Autodesk Inventor part; units mm, degrees
ref_plane "YZ Plane" through (0, 0, 0) normal (1, 0, 0) x (0, 1, 0)
ref_plane "XZ Plane" through (0, 0, 0) normal (0, 1, 0) x (-1, 0, 0)
ref_plane "XY Plane" through (0, 0, 0) normal (0, 0, 1) x (1, 0, 0)
sketch "Sketch1" plane through (0, 0, 0) normal (0, 0, 1) x (1, 0, 0)
  line L0 (34.925, 0) -> (34.925, 12.7)
  arc A0 (34.925, 53.1813) -> (0, 76.2) centre (2.0699, 41.3364) ccw
  line L1 (2.0699, 41.3364) -> (34.925, 53.1813) construction
  spline S0 degree 4 poles (34.925, 53.1812) (39.0776, 41.6628) (-1.6968, 40.738) (-5.8394, 15.6518) (34.925, 23.1641) (34.925, 12.7) knots 0 0 0 0 0 0.508926 1 1 1 1 1
  line L2 (34.925, 0) -> (0, 0)
  line L3 (0, 76.2) -> (0, 0)
  line L4 (6.4324, 32.095) -> (6.2676, 25.055) construction
  point P0 (6.35, 28.575)
  point P1 (10.076, 28.4878)
  point P2 (7.1561, 30.8039)
  point P3 (7.0327, 26.3053)
  dimension "d0" = 34.925
  dimension "d2" = 12.7
  dimension "d5" = 76.2
  dimension "d7" = 34.925
  dimension "d8" = 6.35
  dimension "d9" = 28.575
  dimension "d10" = 40.4813
revolve "Revolution1" add sketch "Sketch1" angle 360 about axis through (34.925, 0, 0) along (-1, 0, 0)
mirror "Mirror1" about plane through (0, 38.1, 0) normal (-1, 0, 0) of "Revolution1"
sketch "Sketch2" plane through (34.925, 0, 0) normal (1, 0, 0) x (0, 0, -1)
  circle A0 centre (0, 0) radius 12.7
  circle A1 centre (0, 0) radius 6.35
  point P0 (0, 12.7)
  dimension "d12" = 12.7
extrude "Extrusion1" cut sketch "Sketch2" against normal through all contours A1
equation "\"d10\" = 0.53125 * d5"
properties part number "Wheel" material "Rubber"
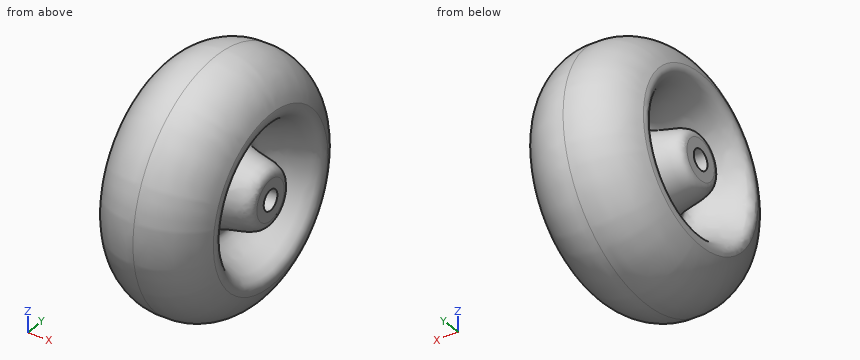
CAD build for the part. Positions are in the model's coordinates, mm. Coordinates: 2 decimals unless noted, no trailing zeros. Write each loop counter-clockwise with the first axis right and the second up, starting at its lowest first coordinate (ties: lowest second). Pieces come first, ordered by that corner, then holes. Notation, with made-up numbers: M 39.5,35.25 L 93.5,35.25 A14 ccw 93.5,42.25 Z; hole C -1,32 d11. An arc over 180 degrees is marked long. Return JSON: item names as keys, results as strings.
Item 1: Drop flat-ended pins along their axis: pin 1 Ø12.5 at (y, z) = (6, -0.5) entering from +X (3 decimals); pin 2 Ø1 at (x, z) = (11, 57.5) entering from +Y; pin 3 Ø6 at (x, z) = (-7.5, 34) entering from +Y. Give the stop position or say it passes through.
Findings below:
{"pin 1": "stops at x = 34.925", "pin 2": "stops at y = 48.93", "pin 3": "stops at y = 69.29"}
Item 2: Slice it at B-B, the plane x = -23.5. State how many separate pieces and enclosed holes the cut face has, and give its area (3 significant figures).
Findings below:
{"separate pieces": "2", "enclosed holes": "2", "area": "10,900 mm2"}
Item 3: Slice it at A-A, the plane x = -3. Write the cut outline in (y, z), and give its area (3 significant figures).
Findings below:
{"outline": "C 0,0 d152.5; hole C 0,0 d12.7", "area": "18,100 mm2"}
Item 4: Probe line 1 (Y direction, x = -9, z = 14); line 2 (Y direction, x = 13, z = 0); line 3 (Y direction, x = -21, z = 0). List the from-to ranges inside material, lowest first. Write a range as from..to.
Findings below:
{"line 1": "y = -74.26..-30.03, -20.21..20.21, 30.03..74.26", "line 2": "y = -74.51..-35.89, -22.89..-6.35, 6.35..22.89, 35.89..74.51", "line 3": "y = -70.69..-39.62, -21.1..-6.35, 6.35..21.1, 39.62..70.69"}
